from build123d import *

# Parameters (mm, degrees)
SKETCH1_R           = 14.2875
BOSS_EXTRUDE1_DEPTH = 7.9248
SKETCH2_R           = 15.5575
SKETCH2_R_2         = 14.2875
BOSS_EXTRUDE2_DEPTH = 1.524


with BuildPart() as part:
    # Sketch1 → Boss-Extrude1 (new body)
    with BuildSketch(Plane(origin=(0, 0, 0), x_dir=(1, 0, 0), z_dir=(0, 1, 0))):
        with Locations(Location((0, 0, 0), (0, 0, 270))):
            Circle(SKETCH1_R)
        Polygon((6.35, -3.666174209), (6.35, 3.666174209), (0, 7.332348419), (-6.35, 3.666174209), (-6.35, -3.666174209), (0, -7.332348419), align=None, mode=Mode.SUBTRACT)
    extrude(amount=BOSS_EXTRUDE1_DEPTH)

    # Sketch2 → Boss-Extrude2 (add)
    with BuildSketch(Plane.XZ):
        with Locations(Location((0, 0, 0), (0, 0, 270))):
            Circle(SKETCH2_R)
        with Locations(Location((0, 0, 0), (0, 0, 270))):
            Circle(SKETCH2_R_2, mode=Mode.SUBTRACT)
    extrude(amount=-BOSS_EXTRUDE2_DEPTH)


solid = part.part
Input: part model. Units: mm. Frame: model coordinates. A direction names the side the tool comes from. Coordinates: 2 decimals unless noted, no trailing zeros. Loops run counter-clockwise (first coordinate to the right, second up) from the corner with the lowest first, then second, coordinate; pieces in that order, holes last.
(1) Section D-D on x = -10.5. Return the cut outline in (y, z).
(2) Section B-B on z = 0. Return the cut outline in (x, y).
(3) Set-up query: faces 5 (the face through (-3.131, 3.907, -5.525)), 6 (the face through (7, 7.925, 0)), 7 (the face through (-13, 1.524, -7)). Return all of +Z, -Z, +X, -X, +Y, -Y with unobstructed straight access to the full face (end or side cutting, diameter ignored); none if empty.
(4) Section C-C on x = 5. Return the cut outline in (y, z).
(5) First-contact query: pin 1 Ø5 at (x, z) = (-3.5, 2) entering from +Y; pin 2 Ø2 at (y, z) = (3, 1) entering from +X; pin 3 Ø1 at (x, y) = (3, 5.5) entering from +Z; pin 4 Ø1 at (x, y) = (7.5, 1) entering from -Z. Flat tips, straight axial feed; report the tip coordinate or a pass-through.
(6) Material intervals for probe 1 along X at (y, z) = (1.75, -1.5); probe 2 along X at (y, z) = (3.5, 6.5); probe 3 along Z at (x, y) = (-6, 5.5), sorted ascending.
(7) Pull-direction query (Z, two-part tool) for faces 1 (the face through (-7, 0, 0)), 2 (the face through (3.219, 3.907, -5.474)), 3 (the face through (4.67, 0.75, -14.84)), 4 (the face through (6.35, 4, 0)); classes: released by +Z, released by -Z, zero draft, split by the parting line, or undercut.
Data:
1. outline: (0, -11.48) - (1.52, -11.48) - (1.52, -9.69) - (7.92, -9.69) - (7.92, 9.69) - (1.52, 9.69) - (1.52, 11.48) - (0, 11.48) - close
2. outline: (-15.56, 0) - (-6.35, 0) - (-6.35, 7.92) - (-14.29, 7.92) - (-14.29, 1.52) - (-15.56, 1.52) - close; (6.35, 0) - (15.56, 0) - (15.56, 1.52) - (14.29, 1.52) - (14.29, 7.92) - (6.35, 7.92) - close
3. face 5: +Y, -Y
3. face 6: +Z, -Z, +X, -X, +Y
3. face 7: +Y
4. outline: (0, -14.73) - (1.52, -14.73) - (1.52, -13.38) - (7.92, -13.38) - (7.92, -4.45) - (0, -4.45) - close; (0, 4.45) - (7.92, 4.45) - (7.92, 13.38) - (1.52, 13.38) - (1.52, 14.73) - (0, 14.73) - close
5. pin 1: passes through
5. pin 2: stops at x = 14.29
5. pin 3: stops at z = 14.07
5. pin 4: stops at z = -13.89
6. probe 1: x = -14.21 to -6.35, 6.35 to 14.21
6. probe 2: x = -12.72 to -1.44, 1.44 to 12.72
6. probe 3: z = -12.97 to -3.87, 3.87 to 12.97
7. face 1: zero draft
7. face 2: undercut
7. face 3: split by the parting line
7. face 4: undercut
